```python
from build123d import *

# Parameters (mm, degrees)
SKETCH1_W           = 228
SKETCH1_H           = 600
SKETCH1_R           = 2.1
SKETCH1_R_2         = 1.6
SKETCH1_W_2         = 100
SKETCH1_H_2         = 340
BOSS_EXTRUDE1_DEPTH = 3.175
FILLET1_R           = 3.2


with BuildPart() as part:
    # Sketch1 → Boss-Extrude1 (new body)
    with BuildSketch(Plane(origin=(0, 0, 0), x_dir=(1, 0, 0), z_dir=(0, 1, 0))):
        Rectangle(SKETCH1_W, SKETCH1_H)
        with Locations(Location((106, 290, 0), (0, 0, 270))):
            Circle(SKETCH1_R, mode=Mode.SUBTRACT)
        with Locations(Location((106, -290, 0), (0, 0, 270))):
            Circle(SKETCH1_R, mode=Mode.SUBTRACT)
        with Locations(Location((78, 290, 0), (0, 0, 90))):
            Circle(SKETCH1_R, mode=Mode.SUBTRACT)
        with Locations(Location((92, 0, 0), (0, 0, 270))):
            Circle(SKETCH1_R_2, mode=Mode.SUBTRACT)
        with Locations(Location((92, 235, 0), (0, 0, 270))):
            Circle(SKETCH1_R_2, mode=Mode.SUBTRACT)
        with Locations(Location((92, -235, 0), (0, 0, 90))):
            Circle(SKETCH1_R_2, mode=Mode.SUBTRACT)
        with Locations(Location((-92, -235, 0), (0, 0, 270))):
            Circle(SKETCH1_R_2, mode=Mode.SUBTRACT)
        with Locations(Location((-106, -290, 0), (0, 0, 90))):
            Circle(SKETCH1_R, mode=Mode.SUBTRACT)
        with Locations(Location((91, -290, 0), (0, 0, 270))):
            Circle(SKETCH1_R, mode=Mode.SUBTRACT)
        with Locations(Location((91, -268, 0), (0, 0, 90))):
            Circle(SKETCH1_R, mode=Mode.SUBTRACT)
        with Locations(Location((106, -268, 0), (0, 0, 90))):
            Circle(SKETCH1_R, mode=Mode.SUBTRACT)
        with Locations(Location((-91, -290, 0), (0, 0, 90))):
            Circle(SKETCH1_R, mode=Mode.SUBTRACT)
        with Locations(Location((-106, -268, 0), (0, 0, 270))):
            Circle(SKETCH1_R, mode=Mode.SUBTRACT)
        with Locations(Location((-91, -268, 0), (0, 0, 270))):
            Circle(SKETCH1_R, mode=Mode.SUBTRACT)
        with Locations(Location((13, -251, 0), (0, 0, 270))):
            Circle(SKETCH1_R, mode=Mode.SUBTRACT)
        with Locations(Location((3, -251, 0), (0, 0, 270))):
            Circle(SKETCH1_R, mode=Mode.SUBTRACT)
        with Locations(Location((13, -211, 0), (0, 0, 90))):
            Circle(SKETCH1_R, mode=Mode.SUBTRACT)
        with Locations(Location((3, -211, 0), (0, 0, 90))):
            Circle(SKETCH1_R, mode=Mode.SUBTRACT)
        with Locations(Location((-39, 290, 0), (0, 0, 270))):
            Circle(SKETCH1_R, mode=Mode.SUBTRACT)
        with Locations(Location((-39, 226.5, 0), (0, 0, 270))):
            Circle(SKETCH1_R, mode=Mode.SUBTRACT)
        with Locations(Location((106, 226.5, 0), (0, 0, 270))):
            Circle(SKETCH1_R, mode=Mode.SUBTRACT)
        with Locations(Location((106, 163, 0), (0, 0, 270))):
            Circle(SKETCH1_R, mode=Mode.SUBTRACT)
        with Locations(Location((106, 99.5, 0), (0, 0, 270))):
            Circle(SKETCH1_R, mode=Mode.SUBTRACT)
        with Locations(Location((106, 36, 0), (0, 0, 270))):
            Circle(SKETCH1_R, mode=Mode.SUBTRACT)
        with Locations(Location((106, -27.5, 0), (0, 0, 270))):
            Circle(SKETCH1_R, mode=Mode.SUBTRACT)
        with Locations(Location((106, -91, 0), (0, 0, 270))):
            Circle(SKETCH1_R, mode=Mode.SUBTRACT)
        with Locations(Location((106, -154.5, 0), (0, 0, 270))):
            Circle(SKETCH1_R, mode=Mode.SUBTRACT)
        with Locations(Location((106, -218, 0), (0, 0, 270))):
            Circle(SKETCH1_R, mode=Mode.SUBTRACT)
        with Locations(Location((78, 226.5, 0), (0, 0, 90))):
            Circle(SKETCH1_R, mode=Mode.SUBTRACT)
        with Locations(Location((78, 163, 0), (0, 0, 90))):
            Circle(SKETCH1_R, mode=Mode.SUBTRACT)
        with Locations(Location((78, 99.5, 0), (0, 0, 90))):
            Circle(SKETCH1_R, mode=Mode.SUBTRACT)
        with Locations(Location((78, 36, 0), (0, 0, 90))):
            Circle(SKETCH1_R, mode=Mode.SUBTRACT)
        with Locations(Location((78, -27.5, 0), (0, 0, 90))):
            Circle(SKETCH1_R, mode=Mode.SUBTRACT)
        with Locations(Location((78, -91, 0), (0, 0, 90))):
            Circle(SKETCH1_R, mode=Mode.SUBTRACT)
        with Locations(Location((78, -154.5, 0), (0, 0, 90))):
            Circle(SKETCH1_R, mode=Mode.SUBTRACT)
        with Locations(Location((78, -218, 0), (0, 0, 90))):
            Circle(SKETCH1_R, mode=Mode.SUBTRACT)
        with Locations(Location((-78, -218, 0), (0, 0, 270))):
            Circle(SKETCH1_R, mode=Mode.SUBTRACT)
        with Locations(Location((-78, -154.5, 0), (0, 0, 270))):
            Circle(SKETCH1_R, mode=Mode.SUBTRACT)
        with Locations(Location((-106, -218, 0), (0, 0, 90))):
            Circle(SKETCH1_R, mode=Mode.SUBTRACT)
        with Locations(Location((-106, -154.5, 0), (0, 0, 90))):
            Circle(SKETCH1_R, mode=Mode.SUBTRACT)
        with Locations(Location((-78, -91, 0), (0, 0, 270))):
            Circle(SKETCH1_R, mode=Mode.SUBTRACT)
        with Locations(Location((-78, -27.5, 0), (0, 0, 270))):
            Circle(SKETCH1_R, mode=Mode.SUBTRACT)
        with Locations(Location((-106, -91, 0), (0, 0, 90))):
            Circle(SKETCH1_R, mode=Mode.SUBTRACT)
        with Locations(Location((-106, -27.5, 0), (0, 0, 90))):
            Circle(SKETCH1_R, mode=Mode.SUBTRACT)
        with Locations(Location((-78, 36, 0), (0, 0, 270))):
            Circle(SKETCH1_R, mode=Mode.SUBTRACT)
        with Locations(Location((-78, 99.5, 0), (0, 0, 270))):
            Circle(SKETCH1_R, mode=Mode.SUBTRACT)
        with Locations(Location((-106, 36, 0), (0, 0, 90))):
            Circle(SKETCH1_R, mode=Mode.SUBTRACT)
        with Locations(Location((-106, 99.5, 0), (0, 0, 90))):
            Circle(SKETCH1_R, mode=Mode.SUBTRACT)
        with Locations(Location((-78, 163, 0), (0, 0, 270))):
            Circle(SKETCH1_R, mode=Mode.SUBTRACT)
        with Locations(Location((-106, 163, 0), (0, 0, 90))):
            Circle(SKETCH1_R, mode=Mode.SUBTRACT)
        with Locations(Location((-78, 226.5, 0), (0, 0, 270))):
            Circle(SKETCH1_R, mode=Mode.SUBTRACT)
        with Locations(Location((-106, 226.5, 0), (0, 0, 90))):
            Circle(SKETCH1_R, mode=Mode.SUBTRACT)
        with Locations(Location((-92, 235, 0), (0, 0, 90))):
            Circle(SKETCH1_R_2, mode=Mode.SUBTRACT)
        with Locations(Location((-106, 290, 0), (0, 0, 90))):
            Circle(SKETCH1_R, mode=Mode.SUBTRACT)
        with Locations(Location((-78, 290, 0), (0, 0, 270))):
            Circle(SKETCH1_R, mode=Mode.SUBTRACT)
        with Locations(Location((-92, 0, 0), (0, 0, 90))):
            Circle(SKETCH1_R_2, mode=Mode.SUBTRACT)
        with Locations(Location((0, 290, 0), (0, 0, 270))):
            Circle(SKETCH1_R, mode=Mode.SUBTRACT)
        with Locations(Location((0, 226.5, 0), (0, 0, 270))):
            Circle(SKETCH1_R, mode=Mode.SUBTRACT)
        with Locations(Location((39, 290, 0), (0, 0, 270))):
            Circle(SKETCH1_R, mode=Mode.SUBTRACT)
        with Locations(Location((39, 226.5, 0), (0, 0, 270))):
            Circle(SKETCH1_R, mode=Mode.SUBTRACT)
        with Locations((0, 30)):
            Rectangle(SKETCH1_W_2, SKETCH1_H_2, mode=Mode.SUBTRACT)
    extrude(amount=BOSS_EXTRUDE1_DEPTH)

    # Fillet1
    fillet1_edges = [part.edges().sort_by_distance(p)[0] for p in [
        (50, 1.5875, 140),
        (50, 1.5875, -200),
        (-50, 1.5875, -200),
        (-50, 1.5875, 140),
        (114, 1.5875, 300),
        (-114, 1.5875, 300),
        (-114, 1.5875, -300),
        (114, 1.5875, -300),
    ]]
    fillet(fillet1_edges, radius=FILLET1_R)


solid = part.part
```
Check sheet for the modelled part. Datum: model origin and axes. Units: mm. Round coordinates to 2 decimals unless told otherwise and drop trailing zeros. Loops run counter-clockwise (first coordinate to the right, second up) from the corner with the lowest first, then second, coordinate; pieces in that order, holes last. Notation, with made-up numbers: (-29, 73) - (-18, 73) arc R34 cw to (-18, 106) - close; hole circle Ø10 at (66, 11.5). An arc over 180 degrees is marked (long way). Answer as a JSON object with one key per item and string values. Group by question number.
Q1. Gauge pin test, flat end, axial feed: P1, Ø6.5, axis at x = 3, z = 251, coming from the +Y side (3 decimals). Record the tip position at first contact, or that the pin passes through.
Q2. Sectioned sample at B-B, the plane y = 1.85. Count the separate pieces of the cut face and the enclosed holes in it, plus the area to 3 significant figures.
Q3. Scan lines: line 1 along Z through (x, y) = (38, 1.35); line 2 along Z through (x, y) = (6.5, 1.8); line 3 along X through (y, z) = (2.05, 59). Record each from-to range of solid material in increasing order. Write a range as [from, to].
Q4. Sectioned sample at A-A, the plane z = 44. Enter the section's corners in (x, y) (3 decimals).
Solution:
{
 "1": {"P1": "stops at y = 3.175"},
 "2": {"separate pieces": "1", "enclosed holes": "61", "area": "102,000 mm²"},
 "3": {"line 1": "z = [-300, -291.85], [-288.15, -228.35], [-224.65, -200], [140, 300]", "line 2": "z = [-300, -200], [140, 300]", "line 3": "x = [-114, -50], [50, 114]"},
 "4": {"outline": "(-114, 0) - (-50, 0) - (-50, 3.175) - (-114, 3.175) - close; (50, 0) - (114, 0) - (114, 3.175) - (50, 3.175) - close"}
}
